from build123d import *

# Parameters (mm, degrees)
F0_W     = 304.8
F0_H     = 76.2
F1_DEPTH = 9.652
F3_DEPTH = 9.653
F5_DEPTH = 25.4
F7_D     = 4


with BuildPart() as f1:
    # F0 (on Top) → F1 (new body)
    with BuildSketch(Plane.XY):
        with Locations((152.4, 38.1)):
            Rectangle(F0_W, F0_H)
    extrude(amount=F1_DEPTH)

    # F2 (on face) → F3 (cut, through all)
    with BuildSketch(Plane.XY.offset(9.652)):
        with BuildLine():
            ThreePointArc((0, 19.111058), (14.444339, 24.101166), (20.574, 38.1))
            ThreePointArc((20.574, 38.1), (14.444339, 52.098834), (0, 57.088942))
            Line((0, 57.088942), (0, 19.111058))
        make_face()
    extrude(amount=-F3_DEPTH, mode=Mode.SUBTRACT)

    # F4 (on face) → F5 (cut)
    with BuildSketch(Plane(origin=(0, 0, 0), x_dir=(1, 0, 0), z_dir=(0, 0, -1))):
        with BuildLine():
            Line((304.8, 0), (36.560555, 0))
            Line((36.560555, 0), (82.587091, -16.752289))
            ThreePointArc((82.587091, -16.752289), (89.002062, -18.471175), (95.618058, -19.05))
            Line((95.618058, -19.05), (304.8, -19.05))
            Line((304.8, -19.05), (304.8, 0))
        make_face()
        with BuildLine():
            Line((304.8, -76.2), (304.8, -57.15))
            Line((304.8, -57.15), (95.618058, -57.15))
            ThreePointArc((95.618058, -57.15), (89.002062, -57.728825), (82.587091, -59.447711))
            Line((82.587091, -59.447711), (36.560555, -76.2))
            Line((36.560555, -76.2), (304.8, -76.2))
        make_face()
    extrude(amount=-F5_DEPTH, mode=Mode.SUBTRACT)

    # F7 (through all)
    with Locations(Plane(origin=(0, 0, 0), x_dir=(1, 0, 0), z_dir=(0, 0, -1))):
        with Locations((6.35, -14.6), (6.35, -61.6)):
            Hole(F7_D / 2)


solid = f1.part
Input: part model. Units: mm. Frame: model coordinates. A direction names the side the tool comes from. Round coordinates to 2 decimals unless told otherwise and drop trailing zeros. Write each loop counter-clockwise with the first axis right and the second up, starting at its lowest first coordinate (ties: lowest second). Pieces come first, ordered by that corner, then holes.
1) Cut plane B-B (x = 199.5). Return the cut outline in (y, z), then the cut area to 3 significant figures.
2) Cut plane A-A (z = 7.5). Return the cut outline in (x, y).
3) Contact query for flat-ended pins moving along their axis: P1, Ø5, axis at x = 190, z = 2.5, coming from the -Y side; P2, Ø1, axis at x = 230.5, z = 5, coming from the +Y side. Output: stop coordinate, or through.
4) Ray query, L1, parallel to Y at x = 6.35, z = 7.5; L2, parallel to Y at x = 280.5, z = 5.5. Return the intervals inside material, ascending.
5) Cut plane C-C (y = 28). Return the cut outline in (x, z), then the cut area to 3 significant figures.
6) Reachability of faces 1 (the flat face through (18, 76.2, 5)), 2 (the flat face through (202, 57.15, 5)), 3 (the flat face through (199, 19.05, 5)) from +Z, -Z, +X, -X, +Y, -Y: full face, straight path, thin tool, end or side. Return the list, or none.
Geometry says:
1. outline: (19.05, 0) - (57.15, 0) - (57.15, 9.65) - (19.05, 9.65) - close
1. area: 368 mm2
2. outline: (0, 0) - (36.56, 0) - (82.59, 16.75) arc R38.1 cw to (95.62, 19.05) - (304.8, 19.05) - (304.8, 57.15) - (95.62, 57.15) arc R38.1 cw to (82.59, 59.45) - (36.56, 76.2) - (0, 76.2) - (0, 57.09) arc R19.05 cw to (20.57, 38.1) arc R19.05 cw to (0, 19.11) - close; hole circle Ø4 at (6.35, 14.6); hole circle Ø4 at (6.35, 61.6)
3. P1: stops at y = 19.05
3. P2: stops at y = 57.15
4. L1: y = 0 to 12.6, 16.6 to 19.67, 56.53 to 59.6, 63.6 to 76.2
4. L2: y = 19.05 to 57.15
5. outline: (17.68, 0) - (304.8, 0) - (304.8, 9.65) - (17.68, 9.65) - close
5. area: 2,770 mm2
6. face 1: +Z, -Z, +X, -X, +Y
6. face 2: +Z, -Z, +X, +Y
6. face 3: +Z, -Z, +X, -Y
